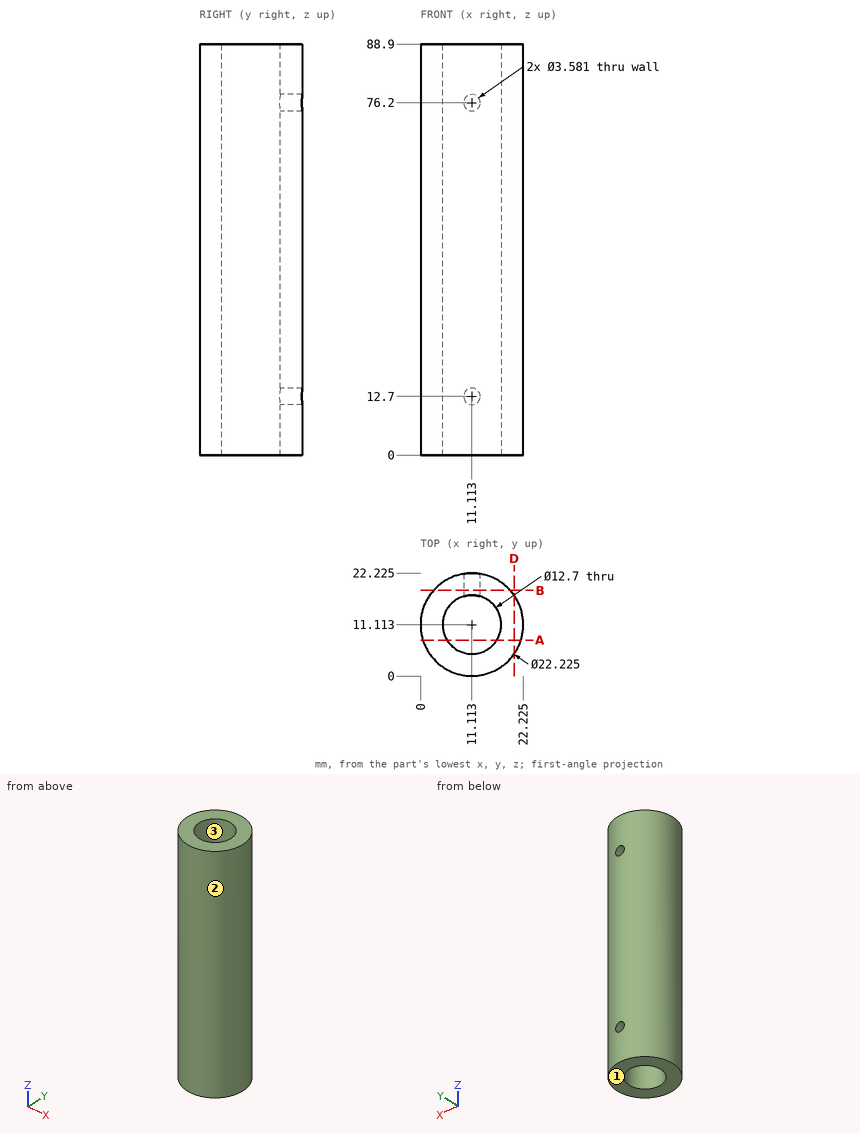
Verification items for this drawing (mm, ordinates from the low corner). Round coordinates to 2 decimals unless told otherwise and drop trailing zeros. Order: outer loops, then holes, each group sorted by start corner. A loop starts at its lowest first (then second) coordinate and runs counter-clockwise, first axis right, second up. Notation, with made-up numbers: M 83.25,-5 L 104.25,-5 A26 cw 104.25,24 Z; hole C -17.75,-26 d6. An arc over 180 degrees is marked long. Answer in a Markdown table with one row per item. Add a question column.
Item 1: Sectioned sample at A-A, the plane y = 7.75. Enter the section's corners in (x, z) (1 decimal).
Item 2: Sectioned sample at B-B, the plane y = 18.5. Enter the section's corners in (x, z).
Item 3: Sectioned sample at D-D, the plane x = 20.25. Enter the section's corners in (y, z).
Item 4: Draft check along X on the marked faces 1, 2 and 3. Enter one of: released by +X, released by -X, zero draft, split by the parting line, or undercut.
Item 5: Material ranges on L1, parallel to X at y = 13.75, z = 13 (1 decimal); L2, parallel to X at y = 6.75, z = 81 (1 decimal); L3, parallel to Y at x = 12, z = 54.5 (1 decimal), recorded low to high. Write a range as [from, to].
Item 6: Depth check by flat-ended pin: pin 1 Ø2 at (x, z) = (6, 73.5) entering from -Y; pin 2 Ø4 at (x, z) = (15, 76) entering from +Y; pin 3 Ø6 at (y, z) = (18, 35) entering from -X; pin 4 Ø10 at (x, y) = (11.11, 11.11) entering from +Z. Enter the tip coordinate at first touch or a pass-through.
Filled in:
| question | item | result |
|---|---|---|
| 1 | outline | M 0.5,0 L 5.7,0 L 5.7,88.9 L 0.5,88.9 Z; M 16.5,0 L 21.7,0 L 21.7,88.9 L 16.5,88.9 Z |
| 2 | outline | M 2.81,0 L 19.41,0 L 19.41,88.9 L 2.81,88.9 Z; hole C 11.11,12.7 d3.58; hole C 11.11,76.2 d3.58 |
| 3 | outline | M 4.79,0 L 17.44,0 L 17.44,88.9 L 4.79,88.9 Z |
| 4 | face 1 | zero draft |
| 4 | face 2 | split by the parting line |
| 4 | face 3 | undercut |
| 5 | L1 | x = [0.3, 5.3], [16.9, 21.9] |
| 5 | L2 | x = [0.9, 6.5], [15.7, 21.3] |
| 5 | L3 | y = [0, 4.8], [17.4, 22.2] |
| 6 | pin 1 | stops at y = 0.79 |
| 6 | pin 2 | stops at y = 22.06 |
| 6 | pin 3 | stops at x = 0.7 |
| 6 | pin 4 | passes through |
